Part model, mm, in its own coordinate system. Face numbers are marked on the shaded views. Coordinates: 2 decimals unless noted, no trailing zeros. Loops run counter-clockwise (first coordinate to the right, second up) from the corner with the lowest first, then second, coordinate; pieces in that order, holes last. Notation, with made-up numbers: (61.5, 27) -> (84.5, 27) arc R13 cw to (84.5, 47) -> close; hole circle Ø10 at (42, -22.75). An arc over 180 degrees is marked (long way). Use one line per item in the form item = value. Start each with the question number.
(1) Drill centre lines: L1, parallel to Y at x = 41, z = 9.5; L2, parallel to Y at x = 41, z = 9.25; L3, parallel to X at y = 16.75, z = 9.5. Where is each one in solid material? Low to high. Write a range as [from, to].
(2) Pin check, flat tip, straight feed: P1, Ø4, axis at y = 7.5, z = 5, coming from the -X side. Stop position of the tip, or through.
(3) Band-saw the part on B-B on x = 4. Give the cut face in (y, z).
(4) Band-saw the part on A-A on z = 1.25. Count the separate pieces of the cut face and the enclosed holes in it, then the cut area to 3 significant figures.
(5) Band-saw the part on D-D on x = 25.5. Give the cut face in (y, z).
(6) Mould opens along Z. For the marked faces 1, 2 and 3 say: +Z half, -Z half, draft (parallel to the pull), parting line (faces both ways), or undercut.
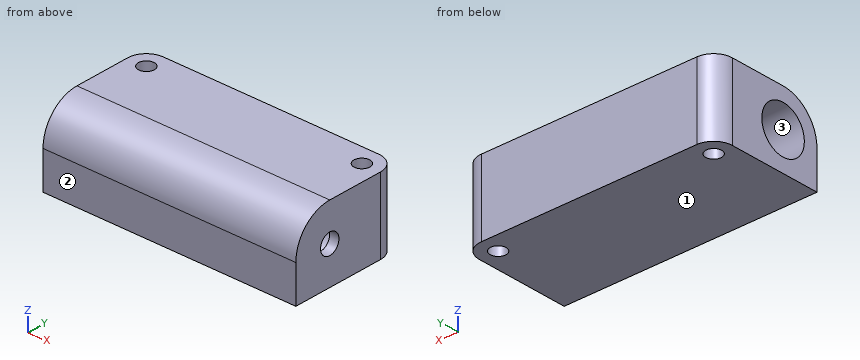
```python
from build123d import *

# Parameters (mm, degrees)
F0_W     = 43.0059846
F0_H     = 19.1125094
F0_R     = 1.35255
F1_DEPTH = 12.7625094
F2_R     = 3.175
F3_R     = 6.3812547
F4_R     = 1.7272
F5_DEPTH = 43.0059846
F6_R     = 4
F6_R_2   = 1.7272
F8_DEPTH = 41.4184846


with BuildPart() as f1:
    # F0 (on Top) → F1 (new body)
    with BuildSketch(Plane.XY):
        with Locations((21.5029923, 9.5562547)):
            Rectangle(F0_W, F0_H)
        with Locations((3.175, 15.9375094)):
            Circle(F0_R, mode=Mode.SUBTRACT)
        with Locations((39.8309846, 15.9375094)):
            Circle(F0_R, mode=Mode.SUBTRACT)
    extrude(amount=F1_DEPTH)

    # F2
    f2_edges = [f1.edges().sort_by_distance(p)[0] for p in [
        (43.005985, 19.112509, 6.381255),
        (0, 19.112509, 6.381255),
    ]]
    fillet(f2_edges, radius=F2_R)

    # F3
    f3_edges = [f1.edges().sort_by_distance(p)[0] for p in [
        (21.502992, 0, 12.762509),
    ]]
    fillet(f3_edges, radius=F3_R)

    # F4 (on face) → F5 (cut, through all)
    with BuildSketch(Plane.YZ.offset(43.0059846)):
        with Locations((6.3812547, 6.3812547)):
            Circle(F4_R)
    extrude(amount=-F5_DEPTH, mode=Mode.SUBTRACT)

    # F6 (on face) → F8 (cut, through all)
    with BuildSketch(Plane(origin=(0, 0, 0), x_dir=(0, -1, 0), z_dir=(-1, 0, 0))):
        with Locations((-6.3812547, 6.3812547)):
            Circle(F6_R)
        with Locations((-6.3812547, 6.3812547)):
            Circle(F6_R_2, mode=Mode.SUBTRACT)
    extrude(amount=-F8_DEPTH, mode=Mode.SUBTRACT)


solid = f1.part
```
A:
q1.L1 = [0.81, 3.88], [8.89, 15.26], [16.62, 18.89]
q1.L2 = [0.68, 3.59], [9.17, 15.26], [16.62, 18.89]
q1.L3 = [0.11, 2.09], [4.26, 38.75], [40.91, 42.9]
q2.P1 = 41.42
q3.outline = (0, 0) -> (14.87, 0) -> (14.87, 12.76) -> (6.38, 12.76) arc R6.38 ccw to (0, 6.38) -> close; (17.01, 0) -> (19.11, 0) -> (19.11, 12.76) -> (17.01, 12.76) -> close; hole circle Ø8 at (6.38, 6.38)
q4.separate_pieces = 1
q4.enclosed_holes = 2
q4.area = 806 mm²
q5.outline = (0, 0) -> (19.11, 0) -> (19.11, 12.76) -> (6.38, 12.76) arc R6.38 ccw to (0, 6.38) -> close; hole circle Ø8 at (6.38, 6.38)
q6.face_1 = -Z half
q6.face_2 = draft
q6.face_3 = undercut
